```python
from build123d import *

# Parameters (mm, degrees)
SKETCH1_W           = 393
SKETCH1_H           = 276
BOSS_EXTRUDE1_DEPTH = 12
SKETCH1_3_R         = 34
CUT_EXTRUDE1_DEPTH  = 12
LPATTERN1_COUNT     = 4
LPATTERN1_PITCH     = 92
SKETCH1_4_R         = 34
CUT_EXTRUDE3_DEPTH  = 12


with BuildPart() as part:
    # Sketch1 → Boss-Extrude1 (new body)
    with BuildSketch(Plane(origin=(0, 0, 0), x_dir=(1, 0, 0), z_dir=(0, 1, 0))):
        with Locations((196.5, 138)):
            Rectangle(SKETCH1_W, SKETCH1_H)
    extrude(amount=BOSS_EXTRUDE1_DEPTH)

    # Sketch1<3> → Cut-Extrude1 (cut)
    with BuildSketch(Plane(origin=(0, 0, 0), x_dir=(1, 0, 0), z_dir=(0, 1, 0))):
        with Locations(Location((46, 46, 0), (0, 0, 270))):
            Circle(SKETCH1_3_R)
        with Locations(Location((46, 230, 0), (0, 0, 270))):
            Circle(SKETCH1_3_R)
    cut_extrude1 = extrude(amount=CUT_EXTRUDE1_DEPTH, mode=Mode.SUBTRACT)

    # LPattern1: Cut-Extrude1 ×4
    with Locations(*[(i * LPATTERN1_PITCH, 0, 0) for i in range(1, LPATTERN1_COUNT)]):
        add(cut_extrude1, mode=Mode.SUBTRACT)

    # Sketch1<4> → Cut-Extrude3 (cut)
    with BuildSketch(Plane(origin=(0, 0, 0), x_dir=(1, 0, 0), z_dir=(0, 1, 0))):
        with BuildLine():
            Line((0, 184), (0, 92))
            Line((0, 92), (77, 92))
            ThreePointArc((77, 92), (87.606601718, 96.393398282), (92, 107))
            Line((92, 107), (92, 169))
            ThreePointArc((92, 169), (87.606601718, 179.606601718), (77, 184))
            Line((77, 184), (0, 184))
        make_face()
        with Locations(Location((138, 138, 0), (0, 0, 90))):
            Circle(SKETCH1_4_R)
        with Locations(Location((322, 138, 0), (0, 0, 90))):
            Circle(SKETCH1_4_R)
    extrude(amount=CUT_EXTRUDE3_DEPTH, mode=Mode.SUBTRACT)


solid = part.part
```
The listing builds one solid part. Answer for the finished solid, in the listing's coordinates (mm). A direction names the side the tool comes from. Give positions to 0.01 mm unless a question says otherwise; leave off trailing zeros. Loops run counter-clockwise (first coordinate to the right, second up) from the corner with the lowest first, then second, coordinate; pieces in that order, holes last. Notation, with made-up numbers: (-11, -25) - (-2, -25) arc R34 ccw to (-2, 12) - close; hole circle Ø9 at (-13.75, 22). An arc over 180 degrees is marked (long way). Return JSON: item names as keys, results as strings. Group by question number.
1. Straight lines are drawn through the part: line 1 (X direction, y = 6.25, z = -230); line 2 (X direction, y = 3.75, z = -138); line 3 (Z direction, x = 133, y = 7.75). For each, find the intervals that lie inside material, in ascending order. Write a range as [from, to].
2. Which of the six approach directions +Z, -Z, +X, -X, +Y, -Y give full straight-line access (tool end or side, diameter ignored) to faces 1 (the cylindrical face through (288.29, 5.92, -133.57)), 2 (the flat face through (38, 6, -92))?
3. Given pin 1 Ø4 at (y, z) = (4, -74) entering from -X, flat-ended and moving along its own axis, determine where the tip first touches the part or whether it passes through.
4. Find section B-B (y = 5.5). State how many separate pieces and enclosed holes the cut face has, then the cut area to 3 significant figures.
5. Find section A-A (x = 230). Write down the section's boundary in (y, z), then the cut area to 3 significant figures.
6. Find section C-C (z = -138). Write down the section's boundary in (x, y), then the cut area to 3 significant figures.
7. Determine the mould class of faces 3 (the flat face through (194, 12, -140)), 4 (the flat face through (194, 6, 0)), 5 (the flat face through (39, 6, -184)) for opening direction Z: pulls with the +Z half, pulls with the -Z half, needs draft (parallel to the pull), parting line crosses it, or undercut.
8. Find section D-D (x = 138). Write down the section's boundary in (y, z), then the cut area to 3 significant figures.
Verdict:
{
 "1": {"line 1": "x = [0, 12], [80, 104], [172, 196], [264, 288], [356, 393]", "line 2": "x = [92, 104], [172, 288], [356, 393]", "line 3": "z = [-276, -263.63], [-196.37, -171.63], [-104.37, -79.63], [-12.37, 0]"},
 "2": {"face 1": "+Y, -Y", "face 2": "-X, +Y, -Y"},
 "3": {"pin 1": "stops at x = 0"},
 "4": {"separate pieces": "1", "enclosed holes": "10", "area": "63,800 mm^2"},
 "5": {"outline": "(0, -276) - (12, -276) - (12, -264) - (0, -264) - close; (0, -196) - (12, -196) - (12, -80) - (0, -80) - close; (0, -12) - (12, -12) - (12, 0) - (0, 0) - close", "area": "1,680 mm^2"},
 "6": {"outline": "(92, 0) - (104, 0) - (104, 12) - (92, 12) - close; (172, 0) - (288, 0) - (288, 12) - (172, 12) - close; (356, 0) - (393, 0) - (393, 12) - (356, 12) - close", "area": "1,980 mm^2"},
 "7": {"face 3": "needs draft", "face 4": "pulls with the +Z half", "face 5": "undercut"},
 "8": {"outline": "(0, -276) - (12, -276) - (12, -264) - (0, -264) - close; (0, -196) - (12, -196) - (12, -172) - (0, -172) - close; (0, -104) - (12, -104) - (12, -80) - (0, -80) - close; (0, -12) - (12, -12) - (12, 0) - (0, 0) - close", "area": "864 mm^2"}
}
